```python
from build123d import *

# Parameters (mm, degrees)
PAD_DEPTH    = 10
FILLET_R     = 1
FILLET001_R  = 1
FILLET002_R  = 1
FILLET003_R  = 1
FILLET004_R  = 1
FILLET005_R  = 1
SKETCH001_R  = 3
POCKET_DEPTH = 5


with BuildPart() as part:
    # Sketch → Pad (new body)
    with BuildSketch(Plane.XY):
        Polygon((10, 0), (10, 70), (60, 70), (60, 60), (20, 60), (20, 0), align=None)
    extrude(amount=PAD_DEPTH)

    # Fillet
    fillet_edges = [part.edges().sort_by_distance(p)[0] for p in [
        (35, 70, 10),
    ]]
    fillet(fillet_edges, radius=FILLET_R)

    # Fillet001
    fillet001_edges = [part.edges().sort_by_distance(p)[0] for p in [
        (35, 70, 0),
    ]]
    fillet(fillet001_edges, radius=FILLET001_R)

    # Fillet002
    fillet002_edges = [part.edges().sort_by_distance(p)[0] for p in [
        (60, 70, 5),
    ]]
    fillet(fillet002_edges, radius=FILLET002_R)

    # Fillet003
    fillet003_edges = [part.edges().sort_by_distance(p)[0] for p in [
        (20, 30, 10),
    ]]
    fillet(fillet003_edges, radius=FILLET003_R)

    # Fillet004
    fillet004_edges = [part.edges().sort_by_distance(p)[0] for p in [
        (20, 30, 0),
    ]]
    fillet(fillet004_edges, radius=FILLET004_R)

    # Fillet005
    fillet005_edges = [part.edges().sort_by_distance(p)[0] for p in [
        (10, 34.5, 10),
    ]]
    fillet(fillet005_edges, radius=FILLET005_R)

    # Sketch001 (on Face1 of Fillet005) → Pocket (cut)
    with BuildSketch(Plane.XZ):
        with Locations((15, 5)):
            Circle(SKETCH001_R)
    extrude(amount=-POCKET_DEPTH, mode=Mode.SUBTRACT)


solid = part.part
```
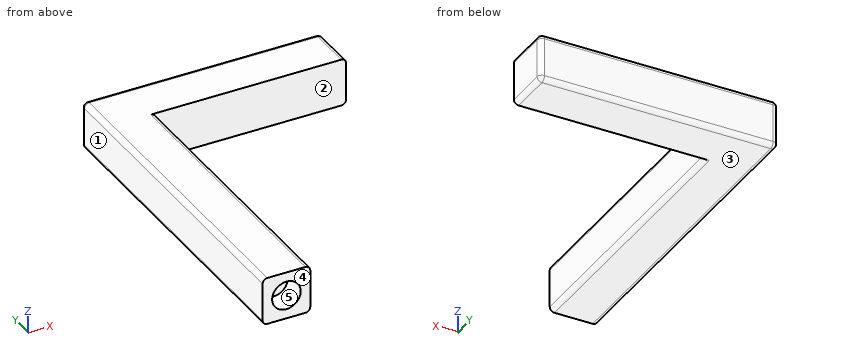
Model file for the job. Use its own axes, mm. Face numbers are marked on the shaded views. A direction names the side the tool comes from. Coordinates: 2 decimals unless noted, no trailing zeros. Loops run counter-clockwise (first coordinate to the right, second up) from the corner with the lowest first, then second, coordinate; pieces in that order, holes last. Notation, with made-up numbers: (59.5, 31) - (96.5, 31) arc R26 ccw to (96.5, 55) - close; hole circle Ø2 at (3.25, -27.5). An arc over 180 degrees is marked (long way). Write item = value, one per line. Start each with the question number.
Item 1: Wall check: probe 1 along Z at (x, y) = (15, 2.4); probe 2 along Y at (x, z) = (54.5, 5); probe 3 along X at (y, z) = (49, 3.75). Give the ranges that are in metal, low to high. Write a range as [from, to].
Item 2: Drop flat-ended pins along their axis: pin 1 Ø5 at (x, z) = (45, 7) entering from -Y; pin 2 Ø2.5 at (y, z) = (27, 4) entering from +X; pin 3 Ø5 at (x, z) = (16, 4) entering from -Y. Give the stop position or say it passes through.
Item 3: Saw through at C-C, the plane z = 5. List the corners of the cut face in (x, y), then the cut area to 3 significant figures.
Item 4: Pull direction Z, two halves, no side cores. Call the marked faces 3, 4 and 5: +Z half, -Z half, draft (parallel to the pull), parting line (faces both ways), or undercut.
Item 5: Saw through at B-B, the plane x = 15. List the corners of the cut face in (y, z), then the cut area to 3 significant figures.
Item 6: Saw through at A-A, the plane y = 15.5. List the corners of the cut face in (x, z).
Item 7: Saw through at D-D, the plane x = 40. List the corners of the cut face in (y, z), then the cut area to 3 significant figures.
Item 8: 3-axis set-ups, long thin cutter, end or side, ignore diameter. For the marked faces 1 and 2: which of +Z, -Z, +X, -X, +Y, -Y reach the whole face in a straight line?
Answers:
q1.probe_1 = [0, 2], [8, 10]
q1.probe_2 = [60, 70]
q1.probe_3 = [10, 20]
q2.pin_1 = 60
q2.pin_2 = 20
q2.pin_3 = 0
q3.outline = (10, 0) - (12, 0) - (12, 5) - (18, 5) - (18, 0) - (20, 0) - (20, 60) - (60, 60) - (60, 69) arc R1 ccw to (59, 70) - (11, 70) arc R1 ccw to (10, 69) - close
q3.area = 1,070 mm2
q4.face_3 = -Z half
q4.face_4 = draft
q4.face_5 = undercut
q5.outline = (0, 0) - (69, 0) arc R1 ccw to (70, 1) - (70, 9) arc R1 ccw to (69, 10) - (0, 10) - (0, 8) - (5, 8) - (5, 2) - (0, 2) - close
q5.area = 670 mm2
q6.outline = (10, 1) arc R1 ccw to (11, 0) - (19, 0) arc R1 ccw to (20, 1) - (20, 9) arc R1 ccw to (19, 10) - (11, 10) arc R1 ccw to (10, 9) - close
q7.outline = (60, 0) - (69, 0) arc R1 ccw to (70, 1) - (70, 9) arc R1 ccw to (69, 10) - (60, 10) - close
q7.area = 99.6 mm2
q8.face_1 = +Z, -Z, -X, +Y, -Y
q8.face_2 = +Z, -Z, +X, -Y
